from build123d import *

# Parameters (mm, degrees)
CUT_EXTRUDE_1_DEPTH = 1.3
CHAMFER_628_SIZE    = 0.1


with BuildPart() as part:
    # 草图1 → 旋转1 (revolve)
    with BuildSketch(Plane(origin=(0, 0, 0), x_dir=(0, 0, -1), z_dir=(1, 0, 0))):
        Polygon((0, 0), (0, 2.84), (3, 2.84), (3, 1.5), (9, 1.5), (9, 0), align=None)
    revolve(axis=Axis((0, 0, -9), (0, 0, 1)))

    # 草图2 → 切除-拉伸1 (cut)
    with BuildSketch(Plane.XY):
        Polygon((0.739008345, 1.28), (-0.739008345, 1.28), (-1.478016689, 0), (-0.739008345, -1.28), (0.739008345, -1.28), (1.478016689, 0), align=None)
    extrude(amount=-CUT_EXTRUDE_1_DEPTH, mode=Mode.SUBTRACT)

    # Chamfer 628
    chamfer_628_edges = [part.edges().sort_by_distance(p)[0] for p in [
        (0, -2.84, 0),
    ]]
    chamfer(chamfer_628_edges, length=CHAMFER_628_SIZE)


solid = part.part
Model file for the job. Use its own axes, mm. A direction names the side the tool comes from. Coordinates: 2 decimals unless noted, no trailing zeros. Order: outer loops, then holes, each group sorted by start corner. A loop starts at its lowest first (then second) coordinate and runs counter-clockwise, first axis right, second up. Notation, with made-up numbers: M -36,-4.5 L -9,-4.5 A36 ccw -9,34.5 Z; hole C 76.25,64.25 d10. An arc over 180 degrees is marked long. Return JSON: item names as keys, results as strings.
1. Saw through at C-C (z = -6). Give the cut face in (x, y).
Ans:
{"outline": "C 0,0 d3"}
2. Flat gauge pins, fed straight in: pin 1 (1.5 mm diameter, centred on x = 1.5, y = 2, fed in from -Z); pin 2 (2 mm diameter, centred on y = -1.5, z = -6.5, fed in from -X). Where does each tip first touch, or does it go through?
Ans:
{"pin 1": "z = -3", "pin 2": "x = -1.41"}
3. Tool access for faces 4 (the face through (1.2, 1.2, -3)), 5 (the face through (0, 0, -9)), 6 (the face through (1.103, -0.649, -0.641)): list every direction of +Z, -Z, +X, -X, +Y, -Y with a clear straight run to the whole face (end or side of a thin tool).
Ans:
{"face 4": "-Z", "face 5": "-Z, +X, -X, +Y, -Y", "face 6": "+Z"}
4. Saw through at B-B (z = -1). Give the cut face in (x, y), and give its area (3 significant figures).
Ans:
{"outline": "C 0,0 d5.68; hole M -1.48,0 L -0.74,-1.28 L 0.74,-1.28 L 1.48,0 L 0.74,1.28 L -0.74,1.28 Z", "area": "19.7 mm^2"}
5. Drill centre lines: probe 1 along Z at (x, y) = (0.8, 0.8); probe 2 along Z at (x, y) = (2.2, -1.45); probe 3 along Y at (x, z) = (0.5, -0.25). Where is each one in solid material? Low to high.
Ans:
{"probe 1": "-9 to -1.3", "probe 2": "-3 to 0", "probe 3": "-2.8 to -1.28, 1.28 to 2.8"}
6. Saw through at A-A (x = 0). Give the cut face in (y, z).
Ans:
{"outline": "M -2.84,-3 L -1.5,-3 L -1.5,-9 L 1.5,-9 L 1.5,-3 L 2.84,-3 L 2.84,-0.1 L 2.74,0 L 1.28,0 L 1.28,-1.3 L -1.28,-1.3 L -1.28,0 L -2.74,0 L -2.84,-0.1 Z"}
7. Pull direction Y, two halves, no side cores. Call faces 1 (the face through (-0.125, -2.837, -1.57)), 2 (the face through (1.2, -1.2, 0)), 3 (the face through (0, -1.28, -1)): +Y half, -Y half, draft (parallel to the pull), parting line (faces both ways), or undercut.
Ans:
{"face 1": "parting line", "face 2": "draft", "face 3": "undercut"}
